```python
from build123d import *

# Parameters (mm, degrees)
CUT_EXTRUDE1_DEPTH      = 39.565038065
CUT_EXTRUDE1_DEPTH_BACK = 39.565038065
SKETCH2_W               = 6.35
SKETCH2_H               = 0.889


with BuildPart() as part:
    # Sketch1 → Revolve1 (revolve)
    with BuildSketch(Plane.XY):
        Polygon((0, 8.636), (0, 3.175), (34.12744, 3.175), (34.12744, 5.588), (30.226, 5.588), (30.226, 9.525), (23.876, 9.525), (23.876, 12.7), (16.002, 12.7), (16.002, 9.525), (9.652, 9.525), (9.652, 8.636), align=None)
    revolve(axis=Axis((34.12744, 0, 0), (-1, 0, 0)))

    # Sketch2 → Cut-Extrude1 (cut, two sides: drawn at the far end of the back side and taken through both)
    with BuildSketch(Plane.XY.offset(-CUT_EXTRUDE1_DEPTH_BACK)):
        with Locations((12.827, 9.0805)):
            Rectangle(SKETCH2_W, SKETCH2_H)
        with Locations((27.051, 9.0805)):
            Rectangle(SKETCH2_W, SKETCH2_H)
    extrude(amount=CUT_EXTRUDE1_DEPTH + CUT_EXTRUDE1_DEPTH_BACK, mode=Mode.SUBTRACT)


solid = part.part
```
The model under review builds one solid part; all positions refer to its coordinate system, in mm. A direction names the side the tool comes from. Round coordinates to 2 decimals unless told otherwise and drop trailing zeros. Order: outer loops, then holes, each group sorted by start corner. A loop starts at its lowest first (then second) coordinate and runs counter-clockwise, first axis right, second up. Notation, with made-up numbers: (52.5, 68.25) -> (78.5, 68.25) arc R19 ccw to (78.5, 104.25) -> close; hole circle Ø11 at (48, 31). An arc over 180 degrees is marked (long way). Use a Markdown table: item, result.
Q1. Mouldability with a two-part tool opening along Y and no side actions: class faces 4 (the cylindrical face through (17.3, -0.69, 3.1)), 5 (the flat face through (27, 8.636, 0)), 6 (the flat face through (34.127, -2.4, 2.4)), 7 (the cylindrical face through (19.88, -2.75, 12.4)) as +Y half, -Y half, draft (parallel to the pull), parting line (faces both ways), or undercut.
Values:
| item | result |
|---|---|
| face 4 | undercut |
| face 5 | +Y half |
| face 6 | draft |
| face 7 | parting line |
Q2. Tool access review of faces 1 (the flat face through (13, 8.636, 0)), 2 (the cylindrical face through (4.758, -1.124, -8.563)), 3 (the flat face through (23.876, 9, 0)): name each direction out of +Z, -Z, +X, -X, +Y, -Y from which nothing blocks a thin tool from reaching the whole face with its end or side.
Values:
| item | result |
|---|---|
| face 1 | +Z, -Z, -X, +Y |
| face 2 | -X |
| face 3 | +X |
Q3. For line 1 (Y direction, x = 13, z = 0) (3 decimals); line 2 (Z direction, x = 17, y = 0) (3 decimals), list the stretches that pass through material, from the lowest coordinate up.
Values:
| item | result |
|---|---|
| line 1 | y = -9.525 to -3.175, 3.175 to 8.636 |
| line 2 | z = -12.7 to -3.175, 3.175 to 12.7 |
Q4. We need section B-B on x = 32. Write out the cut boundary in (y, z) (3 decimals).
Values:
| item | result |
|---|---|
| outline | circle Ø11.176 at (0, 0); hole circle Ø6.35 at (0, 0) |
Q5. We need section A-A on y = 0. Write out the cut boundary in (x, z) (3 decimals), then the cut area to 3 significant figures.
Values:
| item | result |
|---|---|
| outline | (0, -8.636) -> (9.652, -8.636) -> (9.652, -9.525) -> (16.002, -9.525) -> (16.002, -12.7) -> (23.876, -12.7) -> (23.876, -9.525) -> (30.226, -9.525) -> (30.226, -5.588) -> (34.127, -5.588) -> (34.127, -3.175) -> (0, -3.175) -> close; (0, 3.175) -> (34.127, 3.175) -> (34.127, 5.588) -> (30.226, 5.588) -> (30.226, 9.525) -> (23.876, 9.525) -> (23.876, 12.7) -> (16.002, 12.7) -> (16.002, 9.525) -> (9.652, 9.525) -> (9.652, 8.636) -> (0, 8.636) -> close |
| area | 436 mm^2 |
Q6. We need section C-C on z = -7.5. Write out the cut boundary in (x, y), then the cut area to 3 significant figures.
Values:
| item | result |
|---|---|
| outline | (0, -4.28) -> (9.65, -4.28) -> (9.65, -5.87) -> (16, -5.87) -> (16, -10.25) -> (23.88, -10.25) -> (23.88, -5.87) -> (30.23, -5.87) -> (30.23, 5.87) -> (23.88, 5.87) -> (23.88, 10.25) -> (16, 10.25) -> (16, 5.87) -> (9.65, 5.87) -> (9.65, 4.28) -> (0, 4.28) -> close |
| area | 393 mm^2 |
Q7. We need section D-D on y = 6.75. Write out the cut boundary in (x, z), then the cut area to 3 significant figures.
Values:
| item | result |
|---|---|
| outline | (0, -5.39) -> (9.65, -5.39) -> (9.65, -6.72) -> (16, -6.72) -> (16, -10.76) -> (23.88, -10.76) -> (23.88, -6.72) -> (30.23, -6.72) -> (30.23, 6.72) -> (23.88, 6.72) -> (23.88, 10.76) -> (16, 10.76) -> (16, 6.72) -> (9.65, 6.72) -> (9.65, 5.39) -> (0, 5.39) -> close |
| area | 444 mm^2 |
Q8. Clearance check with flat-ended pins moving along their axes: P1, Ø5.5, axis at y = 0, z = 0, coming from the +X side; P2, Ø8, axis at x = 28, y = 3, coming from the -Z side (3 decimals); P3, Ø6, axis at x = 10, y = 10, coming from the +Z side; P4, Ø1.9, axis at x = 27, z = 2, coming from the +Y side. State where each tip first meets the part, or that it passes through.
Values:
| item | result |
|---|---|
| P1 | passes through |
| P2 | stops at z = -9.525 |
| P3 | stops at z = 6.46 |
| P4 | stops at y = 8.64 |
